The model under review builds one solid part; all positions refer to its coordinate system, in mm. Face numbers are marked on the shaded views. Coordinates: 2 decimals unless noted, no trailing zeros. Loops run counter-clockwise (first coordinate to the right, second up) from the corner with the lowest first, then second, coordinate; pieces in that order, holes last. Notation, with made-up numbers: M 29.5,79.25 L 58.5,79.25 A9 ccw 58.5,84.25 Z; hole C -14,61 d3. An arc over 180 degrees is marked long. One line per item, written item: value.
```python
from build123d import *

# Parameters (mm, degrees)
SKETCH1_W           = 115
SKETCH1_H           = 102
BOSS_EXTRUDE1_DEPTH = 4
SKETCH11_W          = 103.5
SKETCH11_H          = 90.5
CUT_EXTRUDE5_DEPTH  = 2
SKETCH16_R          = 2.25
CUT_EXTRUDE7_DEPTH  = 13
BOSS_EXTRUDE4_DEPTH = 70


with BuildPart() as part:
    # Sketch1 → Boss-Extrude1 (new body)
    with BuildSketch(Plane(origin=(0, 0, 0), x_dir=(1, 0, 0), z_dir=(0, 1, 0))):
        with Locations((57.5, 51)):
            Rectangle(SKETCH1_W, SKETCH1_H)
    extrude(amount=BOSS_EXTRUDE1_DEPTH)

    # Sketch11 → Cut-Extrude5 (cut)
    with BuildSketch(Plane(origin=(0, 4, 0), x_dir=(1, 0, 0), z_dir=(0, 1, 0))):
        with Locations((57.5, 51)):
            Rectangle(SKETCH11_W, SKETCH11_H)
    extrude(amount=-CUT_EXTRUDE5_DEPTH, mode=Mode.SUBTRACT)

    # Sketch16 → Cut-Extrude7 (cut)
    with BuildSketch(Plane(origin=(0, 2, 0), x_dir=(1, 0, 0), z_dir=(0, 1, 0))):
        with Locations(Location((13, 11, 0), (0, 0, 270))):
            Circle(SKETCH16_R)
        with Locations(Location((13, 91, 0), (0, 0, 270))):
            Circle(SKETCH16_R)
        with Locations(Location((102, 91, 0), (0, 0, 270))):
            Circle(SKETCH16_R)
        with Locations(Location((102, 11, 0), (0, 0, 270))):
            Circle(SKETCH16_R)
    extrude(amount=-CUT_EXTRUDE7_DEPTH, mode=Mode.SUBTRACT)

    # Sketch6 → Boss-Extrude4 (add)
    with BuildSketch(Plane(origin=(0, 4, 0), x_dir=(1, 0, 0), z_dir=(0, 1, 0))):
        Polygon((0, 0), (0, 8), (4, 8), (4, 4), (8, 4), (8, 0), align=None)
        Polygon((107, 0), (115, 0), (115, 8), (111, 8), (111, 4), (107, 4), align=None)
        Polygon((107, 102), (115, 102), (115, 94), (111, 94), (111, 98), (107, 98), align=None)
        Polygon((8, 102), (0, 102), (0, 94), (4, 94), (4, 98), (8, 98), align=None)
    extrude(amount=BOSS_EXTRUDE4_DEPTH)


solid = part.part
```
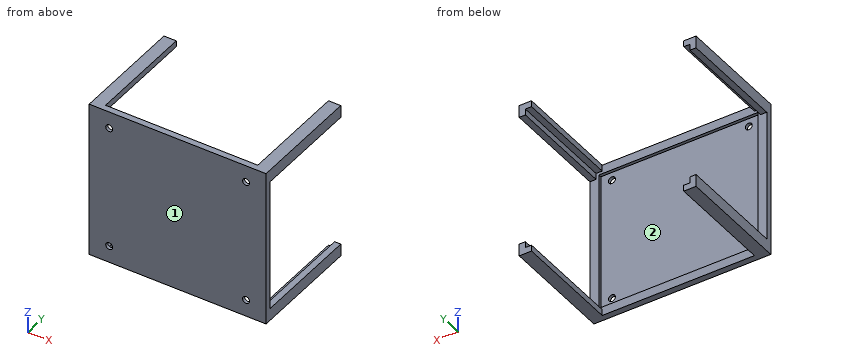
(1) To check wall thickness, follow L1, parallel to X at y = 1.5, z = -91; L2, parallel to Z at x = 110, y = 6; L3, parallel to Y at x = 9, z = -43.5. State the ranges of each line that lie inside material, in increasing order. Write a range as [from, to].
Checks:
L1: [0, 10.75], [15.25, 99.75], [104.25, 115]
L2: [-102, -98], [-4, 0]
L3: [0, 2]
(2) Add section A-A on z = -11. State the section outline as (x, y) points, then the cut area to 3 significant figures.
Checks:
outline: M 0,0 L 10.75,0 L 10.75,2 L 5.75,2 L 5.75,4 L 0,4 Z; M 15.25,0 L 99.75,0 L 99.75,2 L 15.25,2 Z; M 104.25,0 L 115,0 L 115,4 L 109.25,4 L 109.25,2 L 104.25,2 Z
area: 235 mm^2
(3) Draft analysis for pull direction X (two halves, no side actions). For the marked faces 1 and 2, state which applies: pulls with the +X half, pulls with the -X half, needs draft (parallel to the pull), parting line crosses it, or undercut.
Checks:
face 1: needs draft
face 2: undercut
(4) Add section C-C on y = 10.5. State the section outline as (x, z) points, then the cut area to 3 significant figures.
Checks:
outline: M 0,-102 L 8,-102 L 8,-98 L 4,-98 L 4,-94 L 0,-94 Z; M 0,-8 L 4,-8 L 4,-4 L 8,-4 L 8,0 L 0,0 Z; M 107,-102 L 115,-102 L 115,-94 L 111,-94 L 111,-98 L 107,-98 Z; M 107,-4 L 111,-4 L 111,-8 L 115,-8 L 115,0 L 107,0 Z
area: 192 mm^2
(5) Add section D-D on x = 69.5. State the section outline as (y, z) points.
Checks:
outline: M 0,-102 L 4,-102 L 4,-96.25 L 2,-96.25 L 2,-5.75 L 4,-5.75 L 4,0 L 0,0 Z
(6) Insertion check: pin 1 Ø0.6 at (x, y) = (53, 3) entering from +Z; pin 2 Ø1.5 at (x, z) = (28.5, -90.5) entering from +Y. Each pin has a flat end and moves straight along its axis. Give the tip position at first contact, or say it passes through.
Checks:
pin 1: z = 0
pin 2: y = 2
(7) Add section B-B on x = 102. State the section outline as (y, z) points, then the cut area to 3 significant figures.
Checks:
outline: M 0,-102 L 4,-102 L 4,-96.25 L 2,-96.25 L 2,-93.25 L 0,-93.25 Z; M 0,-88.75 L 2,-88.75 L 2,-13.25 L 0,-13.25 Z; M 0,-8.75 L 2,-8.75 L 2,-5.75 L 4,-5.75 L 4,0 L 0,0 Z
area: 209 mm^2
